The listing builds one solid part. Answer for the finished solid, in the listing's coordinates (mm). A direction names the side the tool comes from. Give positions to 0.01 mm unless a question says otherwise; leave off trailing zeros. Loops run counter-clockwise (first coordinate to the right, second up) from the corner with the lowest first, then second, coordinate; pieces in that order, holes last. Notation, with made-up numbers: M -9.5,30 L 37.5,30 A8 cw 37.5,41 Z; hole C 68,69.5 d10. An arc over 180 degrees is marked long. One line per item, written item: value. Start each with the question number.
Q1. A cutting plane is placed at B-B, the plane z = 61. Determine the outline of the cut face in (x, y).
Q2. The mould has two halves that part along Y. Classify faces 1 (the flat face through (-123, 159.762, 91)), 2 (the cylindrical face through (-122.791, 173.106, 174.359)), 3 (the flat face through (-110.268, 158, 84)): +Y half, -Y half, draft (parallel to the pull), parting line (faces both ways), or undercut.
Q3. A cutting plane is placed at A-A, the plane x = -123. Determine the outline of the cut face in (y, z), and give its area (3 significant figures).
Q4. A cutting plane is placed at C-C, the plane y = 222.5. Determine the outline of the cut face in (x, z), and give its area (3 significant figures).
Q5. Consider L1, parallel to Z at x = -124.75, y = 164.5; L2, parallel to Y at x = -126.5, z = 103.5; L3, parallel to Y at x = -116.75, z = 110. Determine where each line is inside the solid, lowest interval first.
Q6. Flat-ended cylindrical pins translate along their axes: pin 1 (1.5 mm diameter, centred on x = -132.5, y = 104, fed in from +Z); pin 2 (3 mm diameter, centred on x = -126.5, y = 155, fed in from +Z); pin 3 (1.8 mm diameter, centred on x = -121, z = 91.5, fed in from -Y). Find the tip coordinate at first contact, or state that the pin passes through.
Q7. For faces 4 (the flat face through (-135.668, 158, 84)), 5 (the flat face through (-123, 153.412, 91)), determine the directions among +Z, -Z, +X, -X, +Y, -Y from which every point of the face is accessible in a straight line to the end or side of a thin tool.
Autodesk Inventor part; units mm, degrees
ref_plane "Work Plane1" through (-110.2685, -72.0125, 201.5707) normal (-1, 0, 0) x (0, -1, 0)
ref_plane "YZ Plane" through (0, 0, 0) normal (1, 0, 0) x (0, 1, 0)
ref_plane "XZ Plane" through (0, 0, 0) normal (0, 1, 0) x (-1, 0, 0)
ref_plane "Work Plane1" through (-110.2685, -72.0125, 201.5707) normal (-1, 0, 0) x (0, -1, 0)
sketch "Sketch1" plane through (-110.2685, -72.0125, 201.5707) normal (-1, 0, 0) x (0, -1, 0)
  circle A0 centre (-228.6, -101.6) radius 12.7
  circle A1 centre (-228.6, -101.6) radius 76.2
  circle A2 centre (-228.6, -101.6) radius 12.7
  point P0 (-72.0125, -201.5707)
  dimension "d0" = 152.4
extrude "Extrusion1" add sketch "Sketch1" along normal blind 25.4
sketch "Sketch4" plane through (-135.6685, 156.5875, 99.9707) normal (-1, 0, 0) x (0, 0, 1)
  circle A0 centre (0, 0) radius 12.7 construction
  line L0 (-12.7, 0) -> (12.7, 0) construction
  line L1 (-6.35, -3.175) -> (-6.35, 3.175)
  line L2 (-6.35, 3.175) -> (-19.05, 3.175)
  line L3 (-19.05, 3.175) -> (-19.05, -3.175)
  line L4 (-19.05, -3.175) -> (-6.35, -3.175)
  line L5 (-6.35, -3.175) -> (-19.05, 3.175) construction
  line L6 (-6.35, 3.175) -> (-19.05, -3.175) construction
  dimension "d7" = 6.35
  dimension "d8" = 12.7
extrude "Extrusion3" add sketch "Sketch4" against normal blind 25.4
properties part number "clutch02-simplyGearDisk" material "PET Plastic"
Answer block:
1. outline: M -135.67,91.11 L -110.27,91.11 L -110.27,222.07 L -135.67,222.07 Z
2. face 1: undercut
2. face 2: parting line
2. face 3: draft
3. outline: C 156.59,99.97 d152.4; hole M 153.41,87.67 L 153.41,93.62 L 159.76,93.62 L 159.76,87.67 A12.7 ccw long Z
3. area: 17,800 mm^2
4. outline: M -135.67,61.73 L -110.27,61.73 L -110.27,138.21 L -135.67,138.21 Z
4. area: 1,940 mm^2
5. L1: 24.18 to 90.04, 109.9 to 175.76
5. L2: 80.47 to 144.39, 168.79 to 232.71
5. L3: 81.05 to 148.8, 164.38 to 232.12
6. pin 1: z = 155.82
6. pin 2: z = 176.17
6. pin 3: y = 80.76
7. face 4: +Z, -Z, -X, +Y, -Y
7. face 5: +X, -X
